from build123d import *

# Parameters (mm, degrees)
SCHIZZO1_R                  = 45
SCHIZZO1_R_2                = 30
ESTRUSIONE1_DEPTH           = 26
SCHIZZO2_R                  = 40.5
SCHIZZO2_R_2                = 32
ESTRUSIONE2_DEPTH           = 10
RIPETIZIONECIRCOLARE1_COUNT = 3
SMUSSO1_SIZE                = 3
SMUSSO2_SIZE                = 1


with BuildPart() as part:
    # Schizzo1 → Estrusione1 (new body)
    with BuildSketch(Plane(origin=(0, 0, 0), x_dir=(1, 0, 0), z_dir=(0, 1, 0))):
        with Locations(Location((0, 0, 0), (0, 0, 90))):
            Circle(SCHIZZO1_R)
        with Locations(Location((0, 0, 0), (0, 0, 90))):
            Circle(SCHIZZO1_R_2, mode=Mode.SUBTRACT)
    extrude(amount=ESTRUSIONE1_DEPTH)

    # Schizzo2 → Estrusione2 (cut)
    with BuildSketch(Plane(origin=(0, 26, 0), x_dir=(1, 0, 0), z_dir=(0, 1, 0))):
        with Locations(Location((0, 0, 0), (0, 0, 270))):
            Circle(SCHIZZO2_R)
        with Locations(Location((0, 0, 0), (0, 0, 270))):
            Circle(SCHIZZO2_R_2, mode=Mode.SUBTRACT)
    extrude(amount=-ESTRUSIONE2_DEPTH, mode=Mode.SUBTRACT)

    # Schizzo3 → Foro filettato M10-1 (revolve, cut)
    with BuildSketch(Plane(origin=(0, 8, 45), x_dir=(0, -1, 0), z_dir=(1, 0, 0))):
        Polygon((0, 0), (0, 50.053657631), (4.25, 47.5), (4.25, 0), align=None)
    foro_filettato_m10_1 = revolve(axis=Axis((0, 8, 51.35), (0, 0, -1)), mode=Mode.SUBTRACT)

    # RipetizioneCircolare1: Foro filettato M10-1 ×3 about axis
    ripetizionecircolare1_axis = Axis((0, 26, 0), (0, -1, 0))
    for i in range(1, RIPETIZIONECIRCOLARE1_COUNT):
        add(foro_filettato_m10_1.rotate(ripetizionecircolare1_axis, i * 360 / RIPETIZIONECIRCOLARE1_COUNT), mode=Mode.SUBTRACT)

    # Smusso1
    smusso1_edges = [part.edges().sort_by_distance(p)[0] for p in [
        (0, 26, 45),
    ]]
    chamfer(smusso1_edges, length=SMUSSO1_SIZE)

    # Smusso2
    smusso2_edges = [part.edges().sort_by_distance(p)[0] for p in [
        (0, 0, 45),
    ]]
    chamfer(smusso2_edges, length=SMUSSO2_SIZE)


solid = part.part
CAD build for the part. Positions are in the model's coordinates, mm. A direction names the side the tool comes from. Coordinates: 2 decimals unless noted, no trailing zeros. Write each loop counter-clockwise with the first axis right and the second up, starting at its lowest first coordinate (ties: lowest second). Pieces come first, ordered by that corner, then holes. Notation, with made-up numbers: M 26.5,82 L 31.5,82 A27 ccw 31.5,100 Z; hole C -15,-33.75 d1. An arc over 180 degrees is marked long. Return JSON: item names as keys, results as strings.
Item 1: Drop flat-ended pins along their axis: pin 1 Ø2 at (x, y) = (11, 22.5) entering from +Z; pin 2 Ø1.5 at (y, z) = (4.5, -30.5) entering from +X; pin 3 Ø4 at (x, y) = (4.5, 20.5) entering from -Z. Give the stop position or say it passes through.
Findings below:
{"pin 1": "stops at z = 43.87", "pin 2": "stops at x = 33.76", "pin 3": "stops at z = -44.93"}
Item 2: Probe line 1 (X direction, y = 22.5, z = 0); line 2 (Y direction, x = 0, z = 40.75); line 3 (Z direction, x = -16.5, y = 19). List the from-to ranges inside material, lowest first. Write a range as from..to.
Findings below:
{"line 1": "x = -45..-40.5, -32..-30, 30..32, 40.5..45", "line 2": "y = 0..3.75, 12.25..26", "line 3": "z = -41.87..-36.99, -27.42..-25.05, 25.05..27.42, 36.99..41.87"}
Item 3: Slice it at C-C, the plane y = 7. Write the cut outline in (x, z).
Findings below:
{"outline": "M -40.87,-18.83 L -27.8,-11.28 A30 cw -4.13,29.71 L -4.13,44.81 A45 ccw Z; M -36.74,-25.98 A45 ccw 36.74,-25.98 L 23.67,-18.43 A30 cw -23.67,-18.43 Z; M 4.13,29.71 A30 cw 27.8,-11.28 L 40.87,-18.83 A45 ccw 4.13,44.81 Z"}
Item 4: Two-plate mould, pull along Z, no slides. Class faces 3 (the cylindrical face through (34.15, 21.07, 21.77)), 4 (the conical face through (16.142, 25.854, -38.932)), 5 (the cylindrical face through (-1.277, 3.946, 37.456)): +Z half, -Z half, draft (parallel to the pull), parting line (faces both ways), or undercut.
Findings below:
{"face 3": "undercut", "face 4": "parting line", "face 5": "draft"}
Item 5: Slice it at B-B, the plane z = 0. Write the cut outline in (x, y), and give its area (3 significant figures).
Findings below:
{"outline": "M -45,1 L -44,0 L -30,0 L -30,26 L -32,26 L -32,16 L -40.5,16 L -40.5,26 L -42,26 L -45,23 Z; M 30,0 L 44,0 L 45,1 L 45,23 L 42,26 L 40.5,26 L 40.5,16 L 32,16 L 32,26 L 30,26 Z", "area": "600 mm2"}
Item 6: Which spindle directions (+Z, -Z, +X, -X, +Y, -Y) get a long thin tool onto all of the face, cutting with end or side? Do faces 1 (the cylindrical face through (-33.249, 4.074, -17.317)), 2 (the cylindrical face through (-31.24, 21.07, -6.94)). Say none if no direction does.
Findings below:
{"face 1": "none", "face 2": "+Y"}
Item 7: Slice it at A-A, the plane x = 0. Write the cut outline in (y, z).
Findings below:
{"outline": "M 0,-44 L 1,-45 L 23,-45 L 26,-42 L 26,-40.5 L 16,-40.5 L 16,-32 L 26,-32 L 26,-30 L 0,-30 Z; M 0,30 L 3.75,30 L 3.75,45 L 1,45 L 0,44 Z; M 12.25,30 L 26,30 L 26,32 L 16,32 L 16,40.5 L 26,40.5 L 26,42 L 23,45 L 12.25,45 Z"}
